Check sheet for the modelled part. Datum: model origin and axes. Units: mm. A direction names the side the tool comes from. Round coordinates to 2 decimals unless told otherwise and drop trailing zeros. Write each loop counter-clockwise with the first axis right and the second up, starting at its lowest first coordinate (ties: lowest second). Pieces come first, ordered by that corner, then holes.
Item 1: Section check D-D, the plane y = -38. Record the cut outline in (x, z), plus the area to 3 significant figures.
Item 2: Section check C-C, the plane x = 84. Record the cut outline in (y, z), plus the area to 3 significant figures.
Item 3: Material ranges on line 1 along X through (y, z) = (-32.5, -24); line 2 along Y through (x, z) = (80.5, 7); line 3 along Z through (x, y) = (97, -25), recorded low to high.
Item 4: Depth check by flat-ended pin: pin 1 (11 mm diameter, centred on x = 105, z = -22, fed in from -Y); pin 2 (3 mm diameter, centred on x = 105.5, z = -15.5, fed in from +Y); pin 3 (6 mm diameter, centred on y = -11.5, z = -28.5, fed in from +X). Enter the tip coordinate at first touch or a pass-through.
Item 5: Section check B-B, the plane z = -19. Record the cut outline in (x, y).
Item 6: Release check for a two-part mould opening along Z. For faces 6 (the flat face through (111, -22, -36.5)), 7 (the flat face through (106, -41.75, -21)), 8 (the flat face through (84, -22, 0.5)), 9 (the flat face through (105, -37, -6)) record: pulls with the +Z half, pulls with the -Z half, needs draft (parallel to the pull), parting line crosses it, or undercut.
Item 7: Set-up check for faces 1 (the flat face through (110, -22, -17)), 2 (the flat face through (84, -2.25, 4)), 3 (the flat face through (105, -7, -6)), 4 (the flat face through (84, -41.75, 4)), 5 (the flat face through (87, -22, 7.5)): record each of +Z, -Z, +X, -X, +Y, -Y from which the full face is reachable in a straight line by a thin tool's end or side.
from build123d import *

# Parameters (mm, degrees)
SKETCH014_W     = 44
SKETCH014_H     = 20
PAD004_DEPTH    = 15
SKETCH015_W     = 39.5
SKETCH015_H     = 11.5
PAD005_DEPTH    = 30.5
SKETCH016_W     = 30
SKETCH016_H     = 7
POCKET005_DEPTH = 41.5
SKETCH017_W     = 39.5
SKETCH017_H     = 10.5
PAD006_DEPTH    = 30.5
SKETCH018_W     = 30
SKETCH018_H     = 7
POCKET006_DEPTH = 44
FILLET006_R     = 5
FILLET007_R     = 3
CHAMFER032_SIZE = 0.3
CHAMFER033_SIZE = 0.5
CHAMFER034_SIZE = 0.3


with BuildPart() as part:
    # Sketch014 → Pad004 (new body)
    with BuildSketch(Plane.YZ):
        Rectangle(SKETCH014_W, SKETCH014_H)
    extrude(amount=PAD004_DEPTH)

    # Sketch015 (on DatumPlane) → Pad005 (join)
    with BuildSketch(Plane(origin=(0, 0, 0), x_dir=(0, 1, 0), z_dir=(-1, 0, 0))):
        Rectangle(SKETCH015_W, SKETCH015_H)
    extrude(amount=PAD005_DEPTH)

    # Sketch016 (on Face11 of Pad005) → Pocket005 (cut)
    with BuildSketch(Plane(origin=(-30.5, 0, 0), x_dir=(0, 1, 0), z_dir=(-1, 0, 0))):
        Rectangle(SKETCH016_W, SKETCH016_H)
    extrude(amount=-POCKET005_DEPTH, mode=Mode.SUBTRACT)

    # Sketch017 (on DatumPlane) → Pad006 (join)
    with BuildSketch(Plane.YX.offset(10)):
        with Locations((0, 7.5)):
            Rectangle(SKETCH017_W, SKETCH017_H)
    extrude(amount=PAD006_DEPTH)

    # Sketch018 (on Face16 of Pad006) → Pocket006 (cut)
    with BuildSketch(Plane.YX.offset(40.5)):
        with Locations((0, 7.5)):
            Rectangle(SKETCH018_W, SKETCH018_H)
    extrude(amount=-POCKET006_DEPTH, mode=Mode.SUBTRACT)

    # Fillet006
    fillet006_edges = [part.edges().sort_by_distance(p)[0] for p in [
        (11, 0, 3.5),
    ]]
    fillet(fillet006_edges, radius=FILLET006_R)

    # Fillet007
    fillet007_edges = [part.edges().sort_by_distance(p)[0] for p in [
        (4, 0, -3.5),
    ]]
    fillet(fillet007_edges, radius=FILLET007_R)

    # Chamfer032
    chamfer032_edges = [part.edges().sort_by_distance(p)[0] for p in [
        (-30.5, 0, -5.75),
        (-30.5, -19.75, 0),
        (-30.5, 19.75, 0),
        (-30.5, 0, 5.75),
        (-30.5, 0, -3.5),
        (-30.5, 15, 0),
        (-30.5, 0, 3.5),
        (-30.5, -15, 0),
        (12.75, 0, -40.5),
        (7.5, -19.75, -40.5),
        (7.5, 19.75, -40.5),
        (2.25, 0, -40.5),
        (11, 0, -40.5),
        (7.5, 15, -40.5),
        (4, 0, -40.5),
        (7.5, -15, -40.5),
    ]]
    chamfer(chamfer032_edges, length=CHAMFER032_SIZE)

    # Chamfer033
    chamfer033_edges = [part.edges().sort_by_distance(p)[0] for p in [
        (7.5, -22, 10),
        (15, -22, 0),
        (7.5, 22, 10),
        (15, 22, 0),
        (15, 0, 10),
    ]]
    chamfer(chamfer033_edges, length=CHAMFER033_SIZE)

    # Chamfer034
    chamfer034_edges = [part.edges().sort_by_distance(p)[0] for p in [
        (-15.1, -19.75, 5.75),
        (-15.1, -19.75, -5.75),
        (-15.1, 19.75, 5.75),
        (-15.1, 19.75, -5.75),
        (2.25, 19.75, -25.1),
        (2.25, -19.75, -25.1),
        (12.75, 19.75, -25.1),
        (12.75, -19.75, -25.1),
    ]]
    chamfer(chamfer034_edges, length=CHAMFER034_SIZE)


with BuildPart() as part_1:
    # Body002 placement: moved
    add(part.part.moved(Location((99, -22, 4))))


solid = part_1.part
Values found:
1. outline: (68.5, -1.45) - (68.8, -1.75) - (99, -1.75) - (99, -6) - (101.25, -6) - (101.25, -36.2) - (101.55, -36.5) - (111.45, -36.5) - (111.75, -36.2) - (111.75, -6) - (114, -6) - (114, 13.5) - (113.5, 14) - (99, 14) - (99, 9.75) - (68.8, 9.75) - (68.5, 9.45) - close
1. area: 971 mm2
2. outline: (-41.75, -1.45) - (-41.45, -1.75) - (-2.55, -1.75) - (-2.25, -1.45) - (-2.25, 9.45) - (-2.55, 9.75) - (-41.45, 9.75) - (-41.75, 9.45) - close; hole (-37, 0.5) - (-7, 0.5) - (-7, 7.5) - (-37, 7.5) - close
2. area: 244 mm2
3. line 1: x = 101.25 to 103, 110 to 111.75
3. line 2: y = -41.75 to -37, -7 to -2.25
3. line 3: z = -1.75 to 0.5, 7.5 to 9.75
4. pin 1: stops at y = -41.75
4. pin 2: stops at y = -2.25
4. pin 3: stops at x = 111.75
5. outline: (101.25, -41.45) - (101.55, -41.75) - (111.45, -41.75) - (111.75, -41.45) - (111.75, -2.55) - (111.45, -2.25) - (101.55, -2.25) - (101.25, -2.55) - close; hole (103, -37) - (110, -37) - (110, -7) - (103, -7) - close
6. face 6: pulls with the -Z half
6. face 7: needs draft
6. face 8: undercut
6. face 9: undercut
7. face 1: -Z
7. face 2: +Z, -Z, -X, +Y
7. face 3: none
7. face 4: +Z, -Z, -X, -Y
7. face 5: -X
